Can you work these out from the model? Positions are in its coordinate system, mm. Coordinates: 2 decimals unless noted, no trailing zeros. Order: outer loops, then holes, each group sorted by start corner. A loop starts at its lowest first (then second) coordinate and runs counter-clockwise, first axis right, second up. Notation, with made-up numbers: (-8.75, 37) -> (22.25, 37) arc R27 ccw to (22.25, 57) -> close; hole circle Ø11 at (45.5, 45.25). An arc over 180 degrees is marked (long way). Write item = value, one per line.
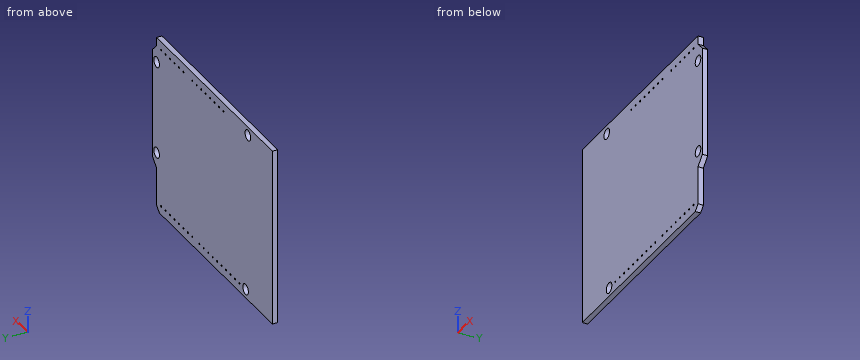
```python
from build123d import *

# Parameters (mm, degrees)
SALIENTE_EXTRUIR1_DEPTH = 1.6002
DRILLS_R                = 1.5875
CORTAR_EXTRUIR1_DEPTH   = 1.6002
PINOUT_R                = 0.254
CORTAR_EXTRUIR2_DEPTH   = 1.6002


with BuildPart() as part:
    # Board → Saliente-Extruir1 (new body)
    with BuildSketch(Plane(origin=(0, 0, 0), x_dir=(1, 0, 0), z_dir=(0, 1, 0))):
        Polygon((68.55, 37.846), (68.55, 5.08), (66.07, 2.54), (66.07, 0), (0, 0), (0, 53.378473106), (64.505207648, 53.378473106), (66.07, 51.813680753), (66.07, 40.386), align=None)
    extrude(amount=SALIENTE_EXTRUIR1_DEPTH)

    # Drills → Cortar-Extruir1 (cut)
    with BuildSketch(Plane(origin=(0, 0, 0), x_dir=(1, 0, 0), z_dir=(0, 1, 0))):
        with Locations(Location((15.27, 50.8, 0), (0, 0, 270))):
            Circle(DRILLS_R)
        with Locations(Location((66.07, 35.56, 0), (0, 0, 270))):
            Circle(DRILLS_R)
        with Locations(Location((66.07, 7.62, 0), (0, 0, 270))):
            Circle(DRILLS_R)
        with Locations(Location((13.970000009, 2.54, 0), (0, 0, 270))):
            Circle(DRILLS_R)
    extrude(amount=CORTAR_EXTRUIR1_DEPTH, mode=Mode.SUBTRACT)

    # Pinout → Cortar-Extruir2 (cut)
    with BuildSketch(Plane(origin=(0, 0, 0), x_dir=(1, 0, 0), z_dir=(0, 1, 0))):
        with Locations(Location((63.50000008, 2.54, 0), (0, 0, 270))):
            Circle(PINOUT_R)
        with Locations(Location((60.96000008, 2.54, 0), (0, 0, 270))):
            Circle(PINOUT_R)
        with Locations(Location((58.42000008, 2.54, 0), (0, 0, 270))):
            Circle(PINOUT_R)
        with Locations(Location((55.88000008, 2.54, 0), (0, 0, 270))):
            Circle(PINOUT_R)
        with Locations(Location((53.34000008, 2.54, 0), (0, 0, 270))):
            Circle(PINOUT_R)
        with Locations(Location((50.80000008, 2.54, 0), (0, 0, 270))):
            Circle(PINOUT_R)
        with Locations(Location((45.72000008, 2.54, 0), (0, 0, 270))):
            Circle(PINOUT_R)
        with Locations(Location((43.18000008, 2.54, 0), (0, 0, 270))):
            Circle(PINOUT_R)
        with Locations(Location((40.64000008, 2.54, 0), (0, 0, 270))):
            Circle(PINOUT_R)
        with Locations(Location((38.10000008, 2.54, 0), (0, 0, 270))):
            Circle(PINOUT_R)
        with Locations(Location((35.56000008, 2.54, 0), (0, 0, 270))):
            Circle(PINOUT_R)
        with Locations(Location((33.02000008, 2.54, 0), (0, 0, 270))):
            Circle(PINOUT_R)
        with Locations(Location((30.48000008, 2.54, 0), (0, 0, 270))):
            Circle(PINOUT_R)
        with Locations(Location((27.94000008, 2.54, 0), (0, 0, 270))):
            Circle(PINOUT_R)
        with Locations(Location((63.50000008, 50.8, 0), (0, 0, 270))):
            Circle(PINOUT_R)
        with Locations(Location((60.96000008, 50.8, 0), (0, 0, 270))):
            Circle(PINOUT_R)
        with Locations(Location((58.42000008, 50.8, 0), (0, 0, 270))):
            Circle(PINOUT_R)
        with Locations(Location((55.88000008, 50.8, 0), (0, 0, 270))):
            Circle(PINOUT_R)
        with Locations(Location((53.34000008, 50.8, 0), (0, 0, 270))):
            Circle(PINOUT_R)
        with Locations(Location((50.80000008, 50.8, 0), (0, 0, 270))):
            Circle(PINOUT_R)
        with Locations(Location((48.26000008, 50.8, 0), (0, 0, 270))):
            Circle(PINOUT_R)
        with Locations(Location((45.72000008, 50.8, 0), (0, 0, 270))):
            Circle(PINOUT_R)
        with Locations(Location((41.68600002, 50.8, 0), (0, 0, 270))):
            Circle(PINOUT_R)
        with Locations(Location((39.14600002, 50.8, 0), (0, 0, 270))):
            Circle(PINOUT_R)
        with Locations(Location((36.60600002, 50.8, 0), (0, 0, 270))):
            Circle(PINOUT_R)
        with Locations(Location((34.06600002, 50.8, 0), (0, 0, 270))):
            Circle(PINOUT_R)
        with Locations(Location((31.52600002, 50.8, 0), (0, 0, 270))):
            Circle(PINOUT_R)
        with Locations(Location((28.98600002, 50.8, 0), (0, 0, 270))):
            Circle(PINOUT_R)
        with Locations(Location((26.44600002, 50.8, 0), (0, 0, 270))):
            Circle(PINOUT_R)
        with Locations(Location((23.90600002, 50.8, 0), (0, 0, 270))):
            Circle(PINOUT_R)
        with Locations(Location((21.36600002, 50.8, 0), (0, 0, 270))):
            Circle(PINOUT_R)
        with Locations(Location((18.82600002, 50.8, 0), (0, 0, 270))):
            Circle(PINOUT_R)
    extrude(amount=CORTAR_EXTRUIR2_DEPTH, mode=Mode.SUBTRACT)


solid = part.part
```
Item 1: I want a section at A-A, the plane z = -7.62. Please give me the cut outline in (x, y).
A:
outline = (0, 0) -> (64.48, 0) -> (64.48, 1.6) -> (0, 1.6) -> close; (67.66, 0) -> (68.55, 0) -> (68.55, 1.6) -> (67.66, 1.6) -> close
Item 2: If I drill on probe 1 along X at (y, z) = (1.25, -7.62); probe 2 along X at (y, z) = (0.9, -35); probe 3 along Z at (x, y) = (65, 0.9), over which ranges is the centre line in solid material (lowest first)?
A:
probe_1 = 0 to 64.48, 67.66 to 68.55
probe_2 = 0 to 64.58, 67.56 to 68.55
probe_3 = -52.88 to -36.73, -34.39 to -8.79, -6.45 to 0
Item 3: I want a section at B-B, the plane y = 1.3. Give the number of separate pieces and of enclosed holes in the cut face, plus the area to 3 significant figures.
A:
separate_pieces = 1
enclosed_holes = 36
area = 3,570 mm2
Item 4: I'm going to push a flat-ended pin straight in: P1, Ø0.5, axis at y = 0.5, z = -44.5, coming from the +X side. Where does the tip first touch, or does it pass through?
A:
P1 = 66.07
